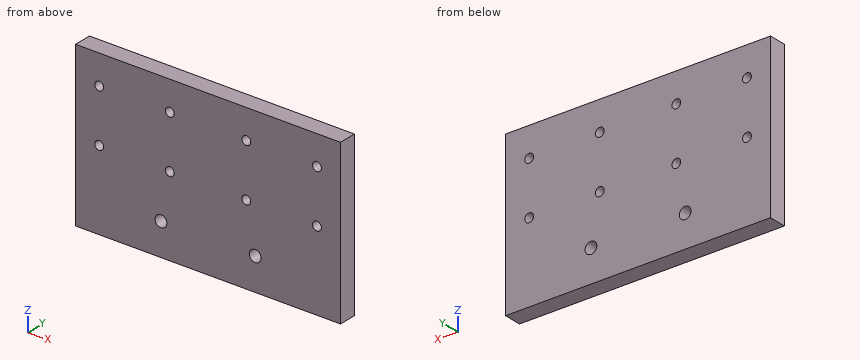
from build123d import *

# Parameters (mm, degrees)
SKETCH1_W           = 90
SKETCH1_H           = 55
SKETCH1_R           = 1.5
BOSS_EXTRUDE1_DEPTH = 6
CUT_EXTRUDE1_REACH  = 8
SKETCH2_R           = 2


with BuildPart() as part:
    # Sketch1 → Boss-Extrude1 (new body)
    with BuildSketch(Plane(origin=(0, 0, 0), x_dir=(1, 0, 0), z_dir=(0, 1, 0))):
        with Locations((0, 2.5)):
            Rectangle(SKETCH1_W, SKETCH1_H)
        with Locations((37, 3)):
            Circle(SKETCH1_R, mode=Mode.SUBTRACT)
        with Locations((13, 3)):
            Circle(SKETCH1_R, mode=Mode.SUBTRACT)
        with Locations((37, -15)):
            Circle(SKETCH1_R, mode=Mode.SUBTRACT)
        with Locations((13, -15)):
            Circle(SKETCH1_R, mode=Mode.SUBTRACT)
        with Locations((-37, -15)):
            Circle(SKETCH1_R, mode=Mode.SUBTRACT)
        with Locations((-37, 3)):
            Circle(SKETCH1_R, mode=Mode.SUBTRACT)
        with Locations((-13, -15)):
            Circle(SKETCH1_R, mode=Mode.SUBTRACT)
        with Locations((-13, 3)):
            Circle(SKETCH1_R, mode=Mode.SUBTRACT)
    extrude(amount=BOSS_EXTRUDE1_DEPTH)

    # Sketch2 → Cut-Extrude1 (cut, up to next)
    with BuildSketch(Plane(origin=(0, 6, 0), x_dir=(1, 0, 0), z_dir=(0, 1, 0)), mode=Mode.PRIVATE) as cut_extrude1_sk1:
        with Locations((16, 19)):
            Circle(SKETCH2_R)
    cut_extrude1_tool1 = extrude(cut_extrude1_sk1.sketch, amount=-CUT_EXTRUDE1_REACH, mode=Mode.PRIVATE) & part.part
    add(cut_extrude1_tool1.solids().sort_by_distance((16, 6, -19))[0], mode=Mode.SUBTRACT)
    # Sketch2 → Cut-Extrude1 (cut, up to next)
    with BuildSketch(Plane(origin=(0, 6, 0), x_dir=(1, 0, 0), z_dir=(0, 1, 0)), mode=Mode.PRIVATE) as cut_extrude1_sk2:
        with Locations((-16, 19)):
            Circle(SKETCH2_R)
    cut_extrude1_tool2 = extrude(cut_extrude1_sk2.sketch, amount=-CUT_EXTRUDE1_REACH, mode=Mode.PRIVATE) & part.part
    add(cut_extrude1_tool2.solids().sort_by_distance((-16, 6, -19))[0], mode=Mode.SUBTRACT)


solid = part.part
Input: part model. Units: mm. Frame: model coordinates. Round coordinates to 2 decimals unless told otherwise and drop trailing zeros. Loops run counter-clockwise (first coordinate to the right, second up) from the corner with the lowest first, then second, coordinate; pieces in that order, holes last. Notation, with made-up numbers: (75, 17.5) -> (83, 17.5) arc R29 ccw to (83, 41.5) -> close; hole circle Ø7 at (32, -30). An arc over 180 degrees is marked (long way). Answer as a JSON object with one key per item and string values. Group by question number.
1) Section query B-B on x = -13. Output: boundary loops of the cut face in (y, z).
2) Pin query (flat end, axial travel): pin 1 (5 mm diameter, centred on x = -13, z = 15, fed in from -Y). Return the tip coordinate at first contact, or that it passes through.
3) Section query A-A on z = -19. Output: boundary loops of the cut face in (x, y).
4) Ray query, L1, parallel to X at y = 3.85, z = 15; L2, parallel to Z at x = 37, y = 3.4; L3, parallel to X at y = 2.65, z = -19. Return the intervals inside material, ascending.
5) Section query D-D on z = 15. Output: boundary loops of the cut face in (x, y).
6) Section query C-C on y = 4. State how many separate pieces and enclosed holes the cut face has, plus the area to 3 significant figures.
Reply:
{
 "1": {"outline": "(0, -30) -> (6, -30) -> (6, -4.5) -> (0, -4.5) -> close; (0, -1.5) -> (6, -1.5) -> (6, 13.5) -> (0, 13.5) -> close; (0, 16.5) -> (6, 16.5) -> (6, 25) -> (0, 25) -> close"},
 "2": {"pin 1": "stops at y = 0"},
 "3": {"outline": "(-45, 0) -> (-18, 0) -> (-18, 6) -> (-45, 6) -> close; (-14, 0) -> (14, 0) -> (14, 6) -> (-14, 6) -> close; (18, 0) -> (45, 0) -> (45, 6) -> (18, 6) -> close"},
 "4": {"L1": "x = -45 to -38.5, -35.5 to -14.5, -11.5 to 11.5, 14.5 to 35.5, 38.5 to 45", "L2": "z = -30 to -4.5, -1.5 to 13.5, 16.5 to 25", "L3": "x = -45 to -18, -14 to 14, 18 to 45"},
 "5": {"outline": "(-45, 0) -> (-38.5, 0) -> (-38.5, 6) -> (-45, 6) -> close; (-35.5, 0) -> (-14.5, 0) -> (-14.5, 6) -> (-35.5, 6) -> close; (-11.5, 0) -> (11.5, 0) -> (11.5, 6) -> (-11.5, 6) -> close; (14.5, 0) -> (35.5, 0) -> (35.5, 6) -> (14.5, 6) -> close; (38.5, 0) -> (45, 0) -> (45, 6) -> (38.5, 6) -> close"},
 "6": {"separate pieces": "1", "enclosed holes": "10", "area": "4,870 mm2"}
}
